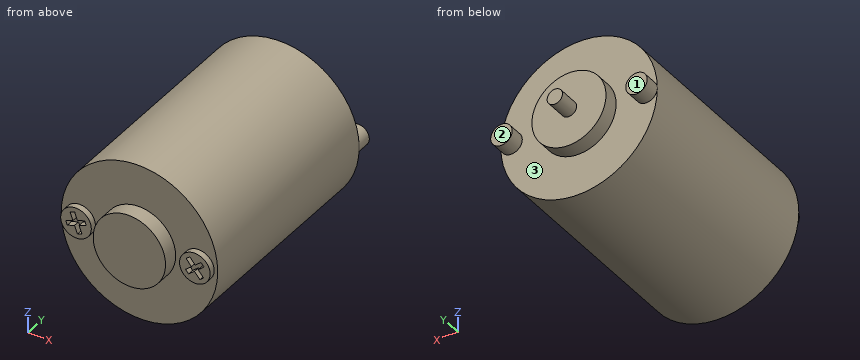
```python
from build123d import *

# Parameters (mm, degrees)
F0_R     = 25.5
F1_DEPTH = 70
F2_R     = 11.791029
F3_DEPTH = 5
F4_R     = 12.078347
F4_R_2   = 3.5
F5_DEPTH = 5
F6_R     = 2.5
F7_DEPTH = 7
F8_R     = 4.991822
F9_DEPTH = 2


with BuildPart() as f1:
    # F0 (on Front) → F1 (new body)
    with BuildSketch(Plane.XZ):
        Circle(F0_R)
    extrude(amount=F1_DEPTH)

    # F2 (on face) → F3 (join)
    with BuildSketch(Plane.XZ.offset(70)):
        Circle(F2_R)
    extrude(amount=F3_DEPTH)

    # F4 (on face) → F5 (join)
    with BuildSketch(Plane(origin=(0, 0, 0), x_dir=(-1, 0, 0), z_dir=(0, 1, 0))):
        Circle(F4_R)
        with Locations((-22, 0)):
            Circle(F4_R_2)
        with Locations((22, 0)):
            Circle(F4_R_2)
    extrude(amount=F5_DEPTH)

    # F6 (on face) → F7 (join)
    with BuildSketch(Plane(origin=(0, 5, 0), x_dir=(-1, 0, 0), z_dir=(0, 1, 0))):
        Circle(F6_R)
    extrude(amount=F7_DEPTH)

    # F8 (on face) → F9 (join)
    with BuildSketch(Plane.XZ.offset(70)):
        with Locations((-19.360058, 0)):
            Circle(F8_R)
        Polygon((-20.359145, 0.43953), (-21.290478, 2.998349), (-19.808572, 3.537719), (-18.877238, 0.9789), (-16.529848, 1.83328), (-16.013582, 0.41485), (-18.360971, -0.43953), (-17.429638, -2.998349), (-18.911544, -3.537719), (-19.842878, -0.9789), (-22.190268, -1.83328), (-22.706534, -0.41485), align=None, mode=Mode.SUBTRACT)
        with Locations((19.360058, 0)):
            Circle(F8_R)
        Polygon((19.241159, -1.085), (17.327549, -2.690709), (16.357286, -1.534394), (18.270895, 0.071316), (16.52056, 2.157284), (17.728622, 3.170968), (19.478957, 1.085), (21.392567, 2.690709), (22.36283, 1.534394), (20.449221, -0.071316), (22.199556, -2.157284), (20.991494, -3.170968), align=None, mode=Mode.SUBTRACT)
    extrude(amount=F9_DEPTH)


solid = f1.part
```
Verification items for the finished model (mm, model axes). Face numbers are marked on the shaded views. A direction names the side the tool comes from. Round coordinates to 2 decimals unless told otherwise and drop trailing zeros. Write each loop counter-clockwise with the first axis right and the second up, starting at its lowest first coordinate (ties: lowest second). Pieces come first, ordered by that corner, then holes.
1. Access from +Z, -Z, +X, -X, +Y, -Y to the whole of each face (thin tool, end or side, straight path). Record for the marked faces 1, 2 and 3.
2. Section check C-C on y = -53. Enter the section's corners in (x, z).
3. Gauge pin test, flat ends, axial feed: P1, Ø3, axis at x = -19, z = -2, coming from the -Y side; P2, Ø5, axis at y = 3, z = 13, coming from the +X side; P3, Ø8, axis at y = -26.5, z = -10.5, coming from the +X side. Record the tip position at first contact, or that the pin passes through.
4. Scan lines: L1, parallel to X at y = -66, z = -1; L2, parallel to Y at x = 10, z = -15; L3, parallel to Y at x = 6, z = 7.5. Record each from-to range of solid material in increasing order.
5. Section check B-B on y = 3. Enter the section's corners in (x, z).
6. Section check A-A on x = 0. Enter the section's corners in (y, z), plus the area to 3 significant figures.
7. Section check D-D on x = -7. Enter the section's corners in (y, z).
Answer:
1. face 1: +Z, -Z, -X, +Y
1. face 2: +Z, -Z, +X, +Y
1. face 3: +Y
2. outline: circle Ø51 at (0, 0)
3. P1: stops at y = -72
3. P2: stops at x = 5.97
3. P3: stops at x = 24.66
4. L1: x = -25.48 to 25.48
4. L2: y = -70 to 0
4. L3: y = -75 to 5
5. outline: circle Ø7 at (-22, 0); circle Ø24.16 at (0, 0); circle Ø7 at (22, 0)
6. outline: (-75, -11.79) - (-70, -11.79) - (-70, -25.5) - (0, -25.5) - (0, -12.08) - (5, -12.08) - (5, -2.5) - (12, -2.5) - (12, 2.5) - (5, 2.5) - (5, 12.08) - (0, 12.08) - (0, 25.5) - (-70, 25.5) - (-70, 11.79) - (-75, 11.79) - close
6. area: 3,840 mm2
7. outline: (-75, -9.49) - (-70, -9.49) - (-70, -24.52) - (0, -24.52) - (0, -9.84) - (5, -9.84) - (5, 9.84) - (0, 9.84) - (0, 24.52) - (-70, 24.52) - (-70, 9.49) - (-75, 9.49) - close
